Build history of the part. All positions in model axes, mm. Give positions to 0.01 mm unless a question says otherwise; leave off trailing zeros. Order: outer loops, then holes, each group sorted by start corner. A loop starts at its lowest first (then second) coordinate and runs counter-clockwise, first axis right, second up. Notation, with made-up numbers: (52, 16) - (75, 16) arc R31 ccw to (75, 49) - close; hole circle Ø8 at (-31.5, 24). An arc over 180 degrees is marked (long way). Answer in a Markdown table with one row per item.
```python
from build123d import *

# Parameters (mm, degrees)
SKETCH1_R           = 14.5542
SKETCH1_R_2         = 2.6289
SKETCH1_R_3         = 3.175
BOSS_EXTRUDE1_DEPTH = 6.35


with BuildPart() as part:
    # Sketch1 → Boss-Extrude1 (new body)
    with BuildSketch(Plane.XY):
        with BuildLine():
            Line((-36.131690566, 5.798452611), (-14.95244478, 33.399783098))
            ThreePointArc((-14.95244478, 33.399783098), (-12.907289703, 35.369766722), (-10.372281426, 36.649308755))
            Line((-10.372281426, 36.649308755), (215.715541799, 111.025764827))
            ThreePointArc((215.715541799, 111.025764827), (222.474160144, 110.71972065), (227.324650683, 106.003225501))
            ThreePointArc((227.324650683, 106.003225501), (242.278345379, 64.918286988), (249.870535149, 21.860839175))
            ThreePointArc((249.870535149, 21.860839175), (248.714513601, 16.416443349), (244.713320148, 12.547556856))
            Line((244.713320148, 12.547556856), (120.65, -50.8))
            Line((120.65, -50.8), (69.85, -50.8))
            Line((69.85, -50.8), (-32.199514598, -8.808434533))
            ThreePointArc((-32.199514598, -8.808434533), (-37.772560831, -2.475984603), (-36.131690566, 5.798452611))
        make_face()
        Circle(SKETCH1_R, mode=Mode.SUBTRACT)
        with Locations((-28.575, 0)):
            Circle(SKETCH1_R_2, mode=Mode.SUBTRACT)
        with Locations((-7.395754214, 27.601330486)):
            Circle(SKETCH1_R_2, mode=Mode.SUBTRACT)
        with Locations((240.38178065, 21.030680725)):
            Circle(SKETCH1_R_3, mode=Mode.SUBTRACT)
        with Locations((233.077901884, 62.453035583)):
            Circle(SKETCH1_R_3, mode=Mode.SUBTRACT)
        with Locations((218.692069012, 101.977786558)):
            Circle(SKETCH1_R_3, mode=Mode.SUBTRACT)
        with Locations((82.55, -38.1)):
            Circle(SKETCH1_R_2, mode=Mode.SUBTRACT)
        with Locations((107.95, -38.1)):
            Circle(SKETCH1_R_2, mode=Mode.SUBTRACT)
        with Locations((25.4, 0)):
            Circle(SKETCH1_R_2, mode=Mode.SUBTRACT)
        with Locations((177.875240911, 47.661527156)):
            Circle(SKETCH1_R_2, mode=Mode.SUBTRACT)
        with Locations((183.141207032, 19.248916511)):
            Circle(SKETCH1_R_2, mode=Mode.SUBTRACT)
    extrude(amount=BOSS_EXTRUDE1_DEPTH)


solid = part.part
```
1. Drop flat-ended pins along their axis: P1, Ø3, axis at y = 15, z = 5, coming from the +X side; P2, Ø6, axis at x = 25.4, y = 0, coming from the -Z side; P3, Ø5.5, axis at x = 233.08, y = 62.45, coming from the +Z side; P4, Ø2, axis at y = 10.5, z = 1.5, coming from the -X side. Give the stop position or say it passes through.
Check result:
| item | result |
|---|---|
| P1 | stops at x = 248.76 |
| P2 | stops at z = 0 |
| P3 | passes through |
| P4 | stops at x = -33.29 |
2. Cut at C-C on y = -23. Write the cut outline in (x, z), and give its area (3 significant figures).
Check result:
| item | result |
|---|---|
| outline | (2.29, 0) - (175.1, 0) - (175.1, 6.35) - (2.29, 6.35) - close |
| area | 1,100 mm² |
3. Cut at A-A on x = 0. Write the cut outline in (y, z).
Check result:
| item | result |
|---|---|
| outline | (-22.06, 0) - (-14.55, 0) - (-14.55, 6.35) - (-22.06, 6.35) - close; (14.55, 0) - (40.06, 0) - (40.06, 6.35) - (14.55, 6.35) - close |
4. Cut at D-D on x = 202. Write the cut outline in (y, z), and give its area (3 significant figures).
Check result:
| item | result |
|---|---|
| outline | (-9.26, 0) - (106.51, 0) - (106.51, 6.35) - (-9.26, 6.35) - close |
| area | 735 mm² |
5. Probe line 1 (X direction, y = 11, z = 0.5); line 2 (Y direction, x = 218, z = 2.5); line 3 (Y direction, x = 84, z = 1.25). List the from-to ranges inside material, lowest first.
Check result:
| item | result |
|---|---|
| line 1 | x = -32.14 to -9.53, 9.53 to 241.68 |
| line 2 | y = -1.09 to 98.88, 105.08 to 111.48 |
| line 3 | y = -50.8 to -40.29, -35.91 to 67.7 |
6. Two-plate mould, pull along X, no slides. Class faces 1 (the face through (222.385, 110.758, 3.131)), 2 (the face through (109.36, -35.88, 3.13)), 3 (the face through (-37.74, -2.59, 3.13)), 4 (the face through (236.01, 61.24, 3.13)): +X half, -X half, draft (parallel to the pull), parting line (faces both ways), or undercut.
Check result:
| item | result |
|---|---|
| face 1 | parting line |
| face 2 | undercut |
| face 3 | -X half |
| face 4 | undercut |
7. Cut at B-B on z = 5. Count the separate pieces of the cut face and the enclosed holes in it, and give its area (3 significant figures).
Check result:
| item | result |
|---|---|
| separate pieces | 1 |
| enclosed holes | 11 |
| area | 27,300 mm² |
